Can you work these out from the model? Positions are in its coordinate system, mm. A direction names the side the tool comes from. Coordinates: 2 decimals unless noted, no trailing zeros. Write each loop counter-clockwise with the first axis right and the second up, starting at its lowest first coordinate (ties: lowest second). Pieces come first, ordered by that corner, then holes. Notation, with made-up numbers: (-7.75, 0) - (15.25, 0) arc R15 cw to (15.25, 7) - close; hole circle Ø7 at (80.5, 54.25). An arc over 180 degrees is marked (long way). Use one line per item in the form item = value. Start each with the question number.
(1) For pin 1 Ø1.5 at (x, z) = (-10.5, 172) entering from -Y; pin 2 Ø6 at (x, z) = (8, 443) entering from +Y; pin 3 Ø1 at (y, z) = (15.5, 92) entering from +X; pin 4 Ø25 at (x, y) = (3, -8) entering from -Z, each with a flat end and sliding along its axis, tell me the tip position at first contact or that it passes through.
(2) On a 3-axis mill with a long thin cutter (end or side, diameter ignored), from which of +Z, -Z, +X, -X, +Y, -Y can I reach the whole of each face in a straight line? I mean faces 1 (the face through (-6, -5, 533.4)), 2 (the face through (-5.05, -3.87, 25.04)), 3 (the face through (0, 0, 0)). Say none if no direction works.
(3) If we section it at A-A on z = 403: Please give me the cut outline in (x, y), then the cut area to 3 significant figures.
(4) If I drill on probe 1 along Z at (x, y) = (-10, -12.5); probe 2 along X at (y, z) = (-0.5, 450); probe 3 along X at (y, z) = (-18, 128.5), over which ranges is the centre line in solid material (lowest first)? Write a range as from..to.
```python
from build123d import *

# Parameters (mm, degrees)
SKETCH1_R           = 25.4
BOSS_EXTRUDE1_DEPTH = 584.2
SKETCH2_OUTSIDE_W   = 170.52
SKETCH2_OUTSIDE_H   = 170.52
SKETCH2_OUTSIDE_R   = 6.361935525
CUT_EXTRUDE1_DEPTH  = 50.8
SKETCH5_OUTSIDE_W   = 170.52
SKETCH5_OUTSIDE_H   = 170.52
SKETCH5_OUTSIDE_R   = 6.377907631
CUT_EXTRUDE4_DEPTH  = 50.8
CUT_EXTRUDE5_DEPTH  = 535.94
CIRPATTERN1_COUNT   = 4


with BuildPart() as part:
    # Sketch1 → Boss-Extrude1 (new body)
    with BuildSketch(Plane.XY):
        Circle(SKETCH1_R)
    extrude(amount=BOSS_EXTRUDE1_DEPTH)

    # Sketch2 outside → Cut-Extrude1 (cut)
    with BuildSketch(Plane.XY):
        Rectangle(SKETCH2_OUTSIDE_W, SKETCH2_OUTSIDE_H)
        Circle(SKETCH2_OUTSIDE_R, mode=Mode.SUBTRACT)
    extrude(amount=CUT_EXTRUDE1_DEPTH, mode=Mode.SUBTRACT)

    # Sketch5 outside → Cut-Extrude4 (cut)
    with BuildSketch(Plane.XY.offset(584.2)):
        Rectangle(SKETCH5_OUTSIDE_W, SKETCH5_OUTSIDE_H)
        Circle(SKETCH5_OUTSIDE_R, mode=Mode.SUBTRACT)
    extrude(amount=-CUT_EXTRUDE4_DEPTH, mode=Mode.SUBTRACT)

    # Sketch13 → Cut-Extrude5 (cut)
    with BuildSketch(Plane.XY.offset(584.2)):
        with BuildLine():
            ThreePointArc((23.648188812, 19.127264814), (13.102061479, 27.448589733), (0, 30.415277302))
            ThreePointArc((0, 30.415277302), (-5.015277302, 25.4), (0, 20.384722698))
            ThreePointArc((0, 20.384722698), (8.781175571, 18.396409298), (15.84933014, 12.819346848))
            ThreePointArc((15.84933014, 12.819346848), (22.902718459, 12.073876495), (23.648188812, 19.127264814))
        make_face()
    cut_extrude5 = extrude(amount=-CUT_EXTRUDE5_DEPTH, mode=Mode.SUBTRACT)

    # CirPattern1: Cut-Extrude5 ×4 about axis
    cirpattern1_axis = Axis((0, 0, 0), (0, 0, 1))
    for i in range(1, CIRPATTERN1_COUNT):
        add(cut_extrude5.rotate(cirpattern1_axis, i * 360 / CIRPATTERN1_COUNT), mode=Mode.SUBTRACT)


solid = part.part
```
Reported:
q1.pin_1 = -17.9
q1.pin_2 = 19.76
q1.pin_3 = 13.8
q1.pin_4 = 0
q2.face_1 = +Z
q2.face_2 = -Z
q2.face_3 = -Z, +X, -X, +Y, -Y
q3.outline = (-24.9, -4.99) arc R25.4 ccw to (-22.5, -11.78) arc R5.02 cw to (-15.85, -12.82) arc R20.38 ccw to (0, -20.38) arc R5.02 cw to (4.99, -24.9) arc R25.4 ccw to (11.78, -22.5) arc R5.02 cw to (12.82, -15.85) arc R20.38 ccw to (20.38, 0) arc R5.02 cw to (24.9, 4.99) arc R25.4 ccw to (22.5, 11.78) arc R5.02 cw to (15.85, 12.82) arc R20.38 ccw to (0, 20.38) arc R5.02 cw to (-4.99, 24.9) arc R25.4 ccw to (-11.78, 22.5) arc R5.02 cw to (-12.82, 15.85) arc R20.38 ccw to (-20.38, 0) arc R5.02 cw to start
q3.area = 1,470 mm2
q4.probe_1 = 50.8..533.4
q4.probe_2 = -20.41..20.38
q4.probe_3 = -9.57..11.27
